from build123d import *

# Parameters (mm, degrees)
F0_W     = 32
F0_H     = 32
F1_DEPTH = 5
F3_DEPTH = 14.5
F4_DEPTH = 2.75
F7_R     = 2.9999901718
F8_DEPTH = 14
F9_R     = 2


with BuildPart() as f1:
    # F0 (on Top) → F1 (new body)
    with BuildSketch(Plane.XY):
        Rectangle(F0_W, F0_H)
        with BuildLine():
            ThreePointArc((-4.5961940777, -6.7175144213), (-6.7175144213, -6.7175144213), (-6.7175144213, -4.5961940777))
            Line((-6.7175144213, -4.5961940777), (1.767766953, 3.8890872965))
            ThreePointArc((1.767766953, 3.8890872965), (3.8890872965, 3.8890872965), (3.8890872965, 1.767766953))
            Line((3.8890872965, 1.767766953), (-4.5961940777, -6.7175144213))
        make_face(mode=Mode.SUBTRACT)
    extrude(amount=F1_DEPTH)

    # F2 (on face) → F3 (join)
    with BuildSketch(Plane.XY.offset(5)):
        Polygon((-16, 16), (-16, 8), (8, 8), (8, -16), (16, -16), (16, 16), align=None)
    extrude(amount=F3_DEPTH)

    # F2 (on face) → F4 (cut)
    with BuildSketch(Plane.XY.offset(5)):
        with BuildLine():
            Line((0.3535533906, 5.3033008589), (-8.1317279836, -3.1819805153))
            ThreePointArc((-8.1317279836, -3.1819805153), (-8.1317279836, -8.1317279836), (-3.1819805153, -8.1317279836))
            Line((-3.1819805153, -8.1317279836), (5.3033008589, 0.3535533906))
            ThreePointArc((5.3033008589, 0.3535533906), (5.3033008589, 5.3033008589), (0.3535533906, 5.3033008589))
        make_face()
        with BuildLine():
            Line((-6.7175144213, -4.5961940777), (1.767766953, 3.8890872965))
            ThreePointArc((1.767766953, 3.8890872965), (3.8890872965, 3.8890872965), (3.8890872965, 1.767766953))
            Line((3.8890872965, 1.767766953), (-4.5961940777, -6.7175144213))
            ThreePointArc((-4.5961940777, -6.7175144213), (-6.7175144213, -6.7175144213), (-6.7175144213, -4.5961940777))
        make_face(mode=Mode.SUBTRACT)
    extrude(amount=-F4_DEPTH, mode=Mode.SUBTRACT)

    # F6: sweep along a path in F6_path
    with BuildLine(Plane(origin=(8, 8, 19.5), x_dir=(0, 1, 0), z_dir=(0, 0, 1))) as f6_path:
        Line((0, 24), (0, 0))
        Line((0, 0), (-24, 0))
    # F5 (on face) → F6 (sweep)
    with BuildSketch(Plane.XZ.offset(16)):
        Polygon((8, 12), (8, 19.5), (5, 19.5), (5, 15), align=None)
    sweep(path=f6_path.line, transition=Transition.RIGHT)

    # F7 (on face) → F8 (cut)
    with BuildSketch(Plane.XY.offset(19.5)):
        with Locations((5, 5)):
            Circle(F7_R)
    extrude(amount=-F8_DEPTH, mode=Mode.SUBTRACT)

    # F9
    f9_edges = [f1.edges().sort_by_distance(p)[0] for p in [
        (16, -16, 9.75),
        (16, 16, 9.75),
        (-16, 16, 9.75),
        (0, 16, 19.5),
        (16, 0, 19.5),
        (-16, -16, 2.5),
    ]]
    fillet(f9_edges, radius=F9_R)


solid = f1.part
Read the model definition and answer for the solid it produces. Units are mm, in the model's axes. A direction names the side the tool comes from. Round coordinates to 2 decimals unless told otherwise and drop trailing zeros. Write each loop counter-clockwise with the first axis right and the second up, starting at its lowest first coordinate (ties: lowest second). Pieces come first, ordered by that corner, then holes. Notation, with made-up numbers: M 42.25,31 L 64.25,31 A34 ccw 64.25,69 Z; hole C 65.5,67 d3. An arc over 180 degrees is marked long. Use a Markdown table: item, result.
1) The part is cut by section B-B (z = 5.75). Write down the section's boundary in (x, y), plus the area to 3 significant figures.
Answers follow:
| item | result |
|---|---|
| outline | M -16,8 L 8,8 L 8,-16 L 14,-16 A2 ccw 16,-14 L 16,14 A2 ccw 14,16 L -14,16 A2 ccw -16,14 Z |
| area | 445 mm2 |
2) The part is cut by section A-A (y = -2.5). Write down the section's boundary in (x, z).
Answers follow:
| item | result |
|---|---|
| outline | M -16,0 L -4.62,0 L -4.62,2.25 L -7.45,2.25 L -7.45,5 L -16,5 Z; M -0.38,0 L 16,0 L 16,17.5 A2 ccw 14,19.5 L 5,19.5 L 5,15 L 8,12 L 8,5 L 2.45,5 L 2.45,2.25 L -0.38,2.25 Z |
3) Straight lines are drawn through the part: line 1 along Z through (x, y) = (-9.5, -7); line 2 along Y through (x, z) = (5, 14); line 3 along Y through (x, z) = (3, 2). For each, find the intervals that lie inside material, in ascending order. Write a range as [from, to].
Answers follow:
| item | result |
|---|---|
| line 1 | z = [0, 5] |
| line 2 | y = [8, 16] |
| line 3 | y = [-16, 0.88], [4.32, 16] |
4) For a pull along Y with two mould halves and no side action, classify faces 4 (the cylindrical face through (15.43, -15.4, 9.61)), 5 (the flat face through (-7, -1, 5)), 6 (the flat face through (-3.83, 1.12, 3.64)) as pulls with the +Y half, pulls with the -Y half, needs draft (parallel to the pull), parting line crosses it, or undercut.
Answers follow:
| item | result |
|---|---|
| face 4 | pulls with the -Y half |
| face 5 | needs draft |
| face 6 | undercut |
5) The part is cut by section D-D (z = 16.5). Write down the section's boundary in (x, y).
Answers follow:
| item | result |
|---|---|
| outline | M -16,5 L 2,5 A3 cw long 5,2 L 5,-16 L 14,-16 A2 ccw 16,-14 L 16,14 A2 ccw 14,16 L -14,16 A2 ccw -16,14 Z |
6) A tool of negligible diameter and unlimited length cuts with its end or side. For faces 1 (the flat face through (-6, 6, 14)), 2 (the flat face through (-7, 5, 17)), 3 (the flat face through (-0.294, -2.415, 1.109)), from which of +Z, -Z, +X, -X, +Y, -Y can it reach the whole face along a straight path? Write none if from no direction.
Answers follow:
| item | result |
|---|---|
| face 1 | -X, -Y |
| face 2 | +Z, -X, -Y |
| face 3 | +Z, -Z |
7) Flat-ended cylindrical pins translate along their axes: pin 1 (3.5 mm diameter, centred on x = 5, y = 5, fed in from +Z); pin 2 (2 mm diameter, centred on y = -8, z = 16, fed in from -X); pin 3 (1 mm diameter, centred on x = -8, z = 10, fed in from -Y). Find the tip coordinate at first contact, or state that the pin passes through.
Answers follow:
| item | result |
|---|---|
| pin 1 | stops at z = 5 |
| pin 2 | stops at x = 5 |
| pin 3 | stops at y = 8 |
8) The part is cut by section C-C (x = -5.5). Write down the section's boundary in (y, z).
Answers follow:
| item | result |
|---|---|
| outline | M -16,0 L -7.15,0 L -7.15,2.25 L -9.15,2.25 L -9.15,5 L -16,5 Z; M -3.38,0 L 16,0 L 16,17.5 A2 ccw 14,19.5 L 5,19.5 L 5,15 L 8,12 L 8,5 L -0.55,5 L -0.55,2.25 L -3.38,2.25 Z |
